Source: CAD feature listing. Evaluate the final solid. Frame: model axes, mm. A direction names the side the tool comes from. Round coordinates to 2 decimals unless told otherwise and drop trailing zeros. Write each loop counter-clockwise with the first axis right and the second up, starting at its lowest first coordinate (ties: lowest second). Pieces come first, ordered by that corner, then holes. Notation, with made-up numbers: M 75.25,33 L 96.25,33 A27 cw 96.25,57 Z; hole C 70,86 d6. An arc over 180 degrees is marked long. Answer in a Markdown table with one row per item. Add a question column.
Item 1: Material intervals for probe 1 along Z at (x, y) = (-3.5, 5.5) (3 decimals); probe 2 along X at (y, z) = (-4.75, -36.5); probe 3 along X at (y, z) = (3.5, 41), sorted ascending.
Item 2: Cut plane B-B on x = -50.5. Return loops of the section in (y, z), and give its area (3 significant figures).
Item 3: Cut plane A-A on z = 0. Return loops of the section in (x, y) (3 decimals).
Item 4: Set-up query: faces 4 (the face through (98.25, -0.09, 15.05)), 5 (the face through (0, 0, -9.525)), 6 (the face through (-89, 0, -2.794)), 7 (the face through (0, 0, 34.234)), 8 (the face through (20, 0, 58.872)). Return all of +Z, -Z, +X, -X, +Y, -Y with unobstructed straight access to the full face (end or side cutting, diameter ignored); none if empty.
Item 5: Contact query for flat-ended pins moving along their axis: pin 1 (6.5 mm diameter, centred on y = -0.5, z = -12.5, fed in from -X); pin 2 (6.5 mm diameter, centred on x = -16.5, y = 0.5, fed in from -Z); pin 3 (4 mm diameter, centred on x = 93.5, y = 0.5, fed in from +Z). Output: stop coordinate, or through.
Item 6: Mould query, pull axis X, two halves, no side actions, for faces 1 (the face through (40.25, -0.09, -41.93)), 2 (the face through (101.243, 0, 2)), 3 (the face through (63, 0, -50.546)). Classes: released by +X, released by -X, zero draft, split by the parting line, or undercut.
from build123d import *

# Parameters (mm, degrees)
F1_DEPTH = 6.35
F2_SIZE2 = 19.05
F2_SIZE  = 19.05
F3_SIZE2 = 19.05
F3_SIZE  = 19.05


# Not quite as in the source:
# - ends of sketch curves that miss each other by under 0.0002 mm in the source are joined


with BuildPart() as f1:
    # F0 (on Front) → F1 (new body, symmetric)
    with BuildSketch(Plane.XZ):
        with BuildLine():
            Line((101.3459994669, -21.8439942511), (75.8431146328, -21.8439942511))
            Line((75.8431146328, -21.8439942511), (75.8431146328, -2.7939942511))
            Line((75.8431146328, -2.7939942511), (101.2431146328, -2.7939942511))
            Line((101.2431146328, -2.7939942511), (101.2431146328, 6.8580057489))
            ThreePointArc((101.2431146328, 6.8580057489), (98.1684202272, 15.1431425742), (90.4331158589, 19.4165843056))
            Line((90.4331158589, 19.4165843056), (70.9499079155, 22.3487064989))
            ThreePointArc((70.9499079155, 22.3487064989), (54.3920764202, 30.184519391), (44.9188305794, 45.8631469058))
            ThreePointArc((44.9188305794, 45.8631469058), (37.9835870307, 55.281692466), (26.8519516779, 58.8724163371))
            Line((26.8519516779, 58.8724163371), (12.8488468359, 58.8724155428))
            Line((12.8488468359, 58.8724155428), (6.2471146328, 34.2344155428))
            Line((6.2471146328, 34.2344155428), (-6.2471205082, 34.2344155428))
            Line((-6.2471205082, 34.2344155428), (-12.848854109, 58.8724148139))
            Line((-12.848854109, 58.8724148139), (-26.8519589509, 58.8724148139))
            ThreePointArc((-26.8519589509, 58.8724148139), (-37.9835941001, 55.2816903113), (-44.9188371145, 45.8631443577))
            ThreePointArc((-44.9188371145, 45.8631443577), (-54.3920820431, 30.1845162803), (-70.9499131167, 22.3487024742))
            Line((-70.9499131167, 22.3487024742), (-90.4331208938, 19.4165791758))
            ThreePointArc((-90.4331208938, 19.4165791758), (-98.1684250197, 15.1431370056), (-101.2431189553, 6.8580000058))
            Line((-101.2431189553, 6.8580000058), (-101.2431189553, -2.7939999942))
            Line((-101.2431189553, -2.7939999942), (-75.8431173272, -2.7939999942))
            Line((-75.8431173272, -2.7939999942), (-75.8431173272, -21.8439985533))
            Line((-75.8431173272, -21.8439985533), (-101.3460021612, -21.844))
            Line((-101.3460021612, -21.844), (-101.3460005331, -50.546))
            Line((-101.3460005331, -50.546), (-45.2120005331, -50.5459968158))
            Line((-45.2120005331, -50.5459968158), (-35.4220414842, -33.5504287171))
            Line((-35.4220414842, -33.5504287171), (-1.0151e-06, -33.5504287171))
            Line((-1.0151e-06, -33.5504287171), (35.4220394539, -33.5504267077))
            Line((35.4220394539, -33.5504267077), (45.2119994669, -50.5459942511))
            Line((45.2119994669, -50.5459942511), (101.3459994669, -50.5459942511))
            Line((101.3459994669, -50.5459942511), (101.3459994669, -21.8439942511))
        make_face()
        with BuildLine():
            Line((-31.7500042241, 9.525), (31.7499957759, 9.525))
            ThreePointArc((31.7499957759, 9.525), (41.2750042241, 4.2241e-06), (31.7500042241, -9.525))
            Line((31.7500042241, -9.525), (-31.7499957759, -9.525))
            ThreePointArc((-31.7499957759, -9.525), (-41.2750042241, -4.2241e-06), (-31.7500042241, 9.525))
        make_face(mode=Mode.SUBTRACT)
    extrude(amount=F1_DEPTH, both=True)

    # F2
    f2_edges = [f1.edges().sort_by_distance(p)[0] for p in [
        (101.345999, 0, -50.545994),
    ]]
    chamfer(f2_edges, length=F2_SIZE, length2=F2_SIZE2)

    # F3
    f3_edges = [f1.edges().sort_by_distance(p)[0] for p in [
        (-101.346001, 0, -50.546),
    ]]
    chamfer(f3_edges, length=F3_SIZE, length2=F3_SIZE2)


solid = f1.part
Results below:
| question | item | result |
|---|---|---|
| 1 | probe 1 | -33.55 to -9.525, 9.525 to 34.234 |
| 1 | probe 2 | -96.34 to -37.12, 37.12 to 96.34 |
| 1 | probe 3 | -46.6 to -8.06, 8.06 to 46.6 |
| 2 | outline | M -6.35,-50.55 L 6.35,-50.55 L 6.35,34.4 L -6.35,34.4 Z |
| 2 | area | 1,080 mm2 |
| 3 | outline | M -101.243,-6.35 L -41.275,-6.35 L -41.275,6.35 L -101.243,6.35 Z; M 41.275,-6.35 L 101.243,-6.35 L 101.243,6.35 L 41.275,6.35 Z |
| 4 | face 4 | +Z, +X, +Y, -Y |
| 4 | face 5 | +Y, -Y |
| 4 | face 6 | -X, +Y, -Y |
| 4 | face 7 | +Z, +Y, -Y |
| 4 | face 8 | +Z, +X, -X, +Y, -Y |
| 5 | pin 1 | x = -75.84 |
| 5 | pin 2 | z = -33.55 |
| 5 | pin 3 | z = 19.21 |
| 6 | face 1 | undercut |
| 6 | face 2 | released by +X |
| 6 | face 3 | zero draft |
